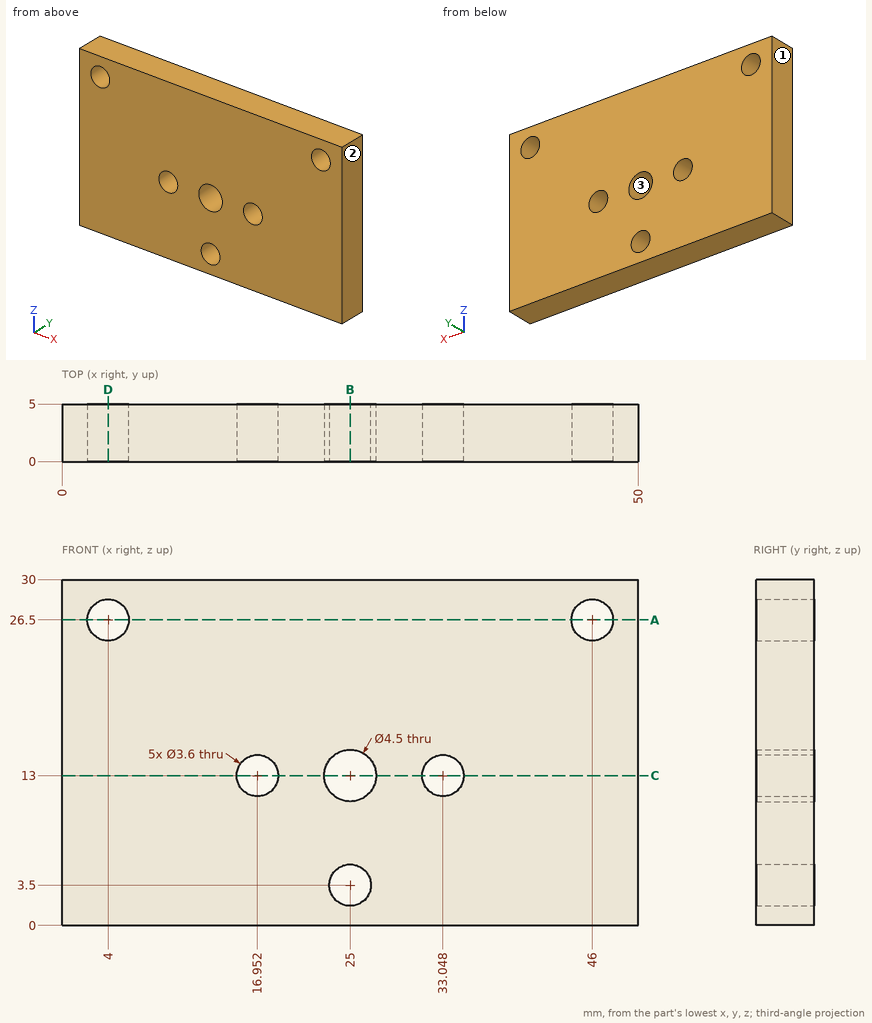
The figure shows three views and two pictorial views of one solid part (mm, origin at its lowest corner). Answer the questions. Round coordinates to 2 decimals unless told otherwise and drop trailing zeros. Write each loop counter-clockwise with the first axis right and the second up, starting at its lowest first coordinate (ties: lowest second). Pieces come first, ordered by that corner, then holes. Notation, with made-up numbers: M 87.25,39.25 L 94.25,39.25 A10 ccw 94.25,55.25 Z; hole C 30,3.25 d4. An arc over 180 degrees is marked long. Use a Markdown table: item, result.
1) The part is cut by section B-B on x = 25. Give the vertices of the cut face in (y, z).
Taken from the geometry:
| item | result |
|---|---|
| outline | M 0,0 L 5,0 L 5,1.7 L 0,1.7 Z; M 0,5.3 L 5,5.3 L 5,10.75 L 0,10.75 Z; M 0,15.25 L 5,15.25 L 5,30 L 0,30 Z |
2) The part is cut by section A-A on z = 26.5. Give the vertices of the cut face in (x, y), plus the area to 3 significant figures.
Taken from the geometry:
| item | result |
|---|---|
| outline | M 0,0 L 2.2,0 L 2.2,5 L 0,5 Z; M 5.8,0 L 44.2,0 L 44.2,5 L 5.8,5 Z; M 47.8,0 L 50,0 L 50,5 L 47.8,5 Z |
| area | 214 mm2 |
3) The part is cut by section D-D on x = 4. Give the vertices of the cut face in (y, z), plus the area to 3 significant figures.
Taken from the geometry:
| item | result |
|---|---|
| outline | M 0,0 L 5,0 L 5,24.7 L 0,24.7 Z; M 0,28.3 L 5,28.3 L 5,30 L 0,30 Z |
| area | 132 mm2 |
4) Consider line 1 (Z direction, x = 25, y = 3.65); line 2 (X direction, y = 2.95, z = 12.5); line 3 (Z direction, x = 4, y = 1.6). Determine where each line is inside the solid, lowest interval first. Write a range as [from, to].
Taken from the geometry:
| item | result |
|---|---|
| line 1 | z = [0, 1.7], [5.3, 10.75], [15.25, 30] |
| line 2 | x = [0, 15.22], [18.68, 22.81], [27.19, 31.32], [34.78, 50] |
| line 3 | z = [0, 24.7], [28.3, 30] |
5) The part is cut by section C-C on z = 13. Give the vertices of the cut face in (x, y), plus the area to 4 significant figures.
Taken from the geometry:
| item | result |
|---|---|
| outline | M 0,0 L 15.15,0 L 15.15,5 L 0,5 Z; M 18.75,0 L 22.75,0 L 22.75,5 L 18.75,5 Z; M 27.25,0 L 31.25,0 L 31.25,5 L 27.25,5 Z; M 34.85,0 L 50,0 L 50,5 L 34.85,5 Z |
| area | 191.5 mm2 |
6) Determine the mould class of the marked faces 1, 2 and 3 for opening direction X: pulls with the +X half, pulls with the -X half, needs draft (parallel to the pull), parting line crosses it, or undercut.
Taken from the geometry:
| item | result |
|---|---|
| face 1 | pulls with the -X half |
| face 2 | pulls with the +X half |
| face 3 | undercut |
